```python
from build123d import *

# Parameters (mm, degrees)
SKETCH1_R           = 2
SKETCH1_W           = 4
SKETCH1_H           = 10
BOSS_EXTRUDE1_DEPTH = 4


with BuildPart() as part:
    # Sketch1 → Boss-Extrude1 (new body)
    with BuildSketch(Plane.XY):
        with BuildLine():
            Line((-30, -19), (-20, -19))
            Line((-20, -19), (-20, -23))
            Line((-20, -23), (-10, -23))
            Line((-10, -23), (-10, -19))
            Line((-10, -19), (10, -19))
            Line((10, -19), (10, -23))
            Line((10, -23), (20, -23))
            Line((20, -23), (20, -19))
            Line((20, -19), (30, -19))
            Line((30, -19), (30, 15))
            ThreePointArc((30, 15), (28.828427125, 17.828427125), (26, 19))
            Line((26, 19), (-26, 19))
            ThreePointArc((-26, 19), (-28.828427125, 17.828427125), (-30, 15))
            Line((-30, 15), (-30, -19))
        make_face()
        with Locations((-10, 0)):
            Circle(SKETCH1_R, mode=Mode.SUBTRACT)
        with Locations((10, 0)):
            Circle(SKETCH1_R, mode=Mode.SUBTRACT)
        with Locations((-24, -1)):
            Rectangle(SKETCH1_W, SKETCH1_H, mode=Mode.SUBTRACT)
        with Locations((24, -1)):
            Rectangle(SKETCH1_W, SKETCH1_H, mode=Mode.SUBTRACT)
    extrude(amount=BOSS_EXTRUDE1_DEPTH)


solid = part.part
```
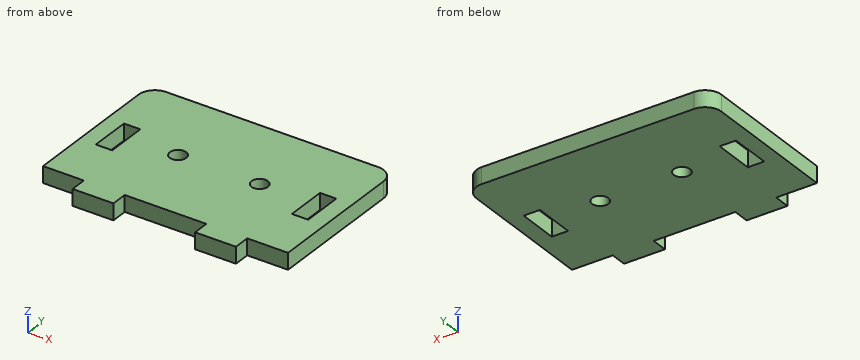
Check sheet for the modelled part. Datum: model origin and axes. Units: mm. Give positions to 0.01 mm unless a question says otherwise; leave off trailing zeros. Write each loop counter-clockwise with the first axis right and the second up, starting at its lowest first coordinate (ties: lowest second). Pieces come first, ordered by that corner, then holes.
Item 1: Cross-section at D-D (x = 5). Enter the section's corners in (y, z).
Item 2: Scan lines: L1, parallel to X at y = -5, z = 0.6; L2, parallel to X at y = -20.5, z = 1.1; L3, parallel to Y at x = -3, z = 1.75. Record each from-to range of solid material in increasing order.
Item 3: Cross-section at A-A (y = 0). Enter the section's corners in (x, z).
Item 4: Gauge pin test, flat ends, axial feed: pin 1 (1.2 mm diameter, centred on x = 23, z = 3, fed in from -Y); pin 2 (6.5 mm diameter, centred on x = -10, y = 0, fed in from +Z); pin 3 (2 mm diameter, centred on y = -21, z = 2, fed in from -X). Record the tip position at first contact, or that the pin passes through.
Item 5: Cross-section at C-C (x = -11). Enter the section's corners in (y, z).
Item 6: Cross-section at B-B (z = 2.3). Enter the section's corners in (x, y).
Report:
1. outline: (-19, 0) - (19, 0) - (19, 4) - (-19, 4) - close
2. L1: x = -30 to -26, -22 to 22, 26 to 30
2. L2: x = -20 to -10, 10 to 20
2. L3: y = -19 to 19
3. outline: (-30, 0) - (-26, 0) - (-26, 4) - (-30, 4) - close; (-22, 0) - (-12, 0) - (-12, 4) - (-22, 4) - close; (-8, 0) - (8, 0) - (8, 4) - (-8, 4) - close; (12, 0) - (22, 0) - (22, 4) - (12, 4) - close; (26, 0) - (30, 0) - (30, 4) - (26, 4) - close
4. pin 1: stops at y = -19
4. pin 2: stops at z = 4
4. pin 3: stops at x = -20
5. outline: (-23, 0) - (-1.73, 0) - (-1.73, 4) - (-23, 4) - close; (1.73, 0) - (19, 0) - (19, 4) - (1.73, 4) - close
6. outline: (-30, -19) - (-20, -19) - (-20, -23) - (-10, -23) - (-10, -19) - (10, -19) - (10, -23) - (20, -23) - (20, -19) - (30, -19) - (30, 15) arc R4 ccw to (26, 19) - (-26, 19) arc R4 ccw to (-30, 15) - close; hole (-26, -6) - (-22, -6) - (-22, 4) - (-26, 4) - close; hole circle Ø4 at (-10, 0); hole circle Ø4 at (10, 0); hole (22, -6) - (26, -6) - (26, 4) - (22, 4) - close
